Autodesk Fusion 360 part; units mm, degrees
sketch "Sketch1" plane through (0, 0, 0) normal (0, 0, 1) x (1, 0, 0)
  circle A0 centre (0, 0) radius 0.975
  dimension "d1" = 1.95
extrude "Extrude1" add sketch "Sketch1" along normal blind 6
sketch "Sketch2" plane through (0, 0, 0) normal (0, 0, -1) x (1, 0, 0)
  circle A0 centre (0, 0) radius 0.975
  circle A1 centre (0, 0) radius 1.75
  dimension "d4" = 3.5
extrude "Extrude2" add sketch "Sketch2" along normal blind 1.5 contours A0 | A1
extrude "Extrude3" cut 1 faces at (-0.5048, -0.8743, -1.5) along direction (0, 0, 1) blind 0.5
equation "d4 = ( 1.75 * 2 ) * 1 mm"
Design review of the part built by this model. Coordinates are the model's own, in mm. A direction names the side the tool comes from. Round coordinates to 2 decimals unless told otherwise and drop trailing zeros. Loops run counter-clockwise (first coordinate to the right, second up) from the corner with the lowest first, then second, coordinate; pieces in that order, holes last. Notation, with made-up numbers: M -33,-37.5 L -25,-37.5 A16 cw -25,-11.5 Z; hole C 5.25,21.25 d8. An arc over 180 degrees is marked long. Answer as a JSON object with one key per item and string values.
Item 1: We need section D-D on y = 1.2. Give the boundary of the cut face in (x, z), and give its area (3 significant figures).
Answer sheet:
{"outline": "M -1.27,-1 L 1.27,-1 L 1.27,0 L -1.27,0 Z", "area": "2.55 mm^2"}
Item 2: We need section A-A on x = 0. Give the boundary of the cut face in (y, z) (3 decimals), and give its area (3 significant figures).
Answer sheet:
{"outline": "M -1.75,-1 L 1.75,-1 L 1.75,0 L 0.975,0 L 0.975,6 L -0.975,6 L -0.975,0 L -1.75,0 Z", "area": "15.2 mm^2"}
Item 3: Machinability: for faces 3 (the cylindrical face through (-0.72, -0.66, 2.96)), 4 (the flat face through (0, 0, -1)), which of the approach directions +Z, -Z, +X, -X, +Y, -Y give a long, thin tool a straight path to every point of the face, cutting with its end or side? Answer none if there is none.
Answer sheet:
{"face 3": "+Z", "face 4": "-Z, +X, -X, +Y, -Y"}
Item 4: We need section C-C on z = 1.5. Give the boundary of the cut face in (x, y) (3 decimals).
Answer sheet:
{"outline": "C 0,0 d1.95"}
Item 5: Clearance check with a flat-ended pin moving along its axis: P1, Ø1.5, axis at x = 1.5, z = 0, coming from the +Y side. State where the tip first meets the part, or that it passes through.
Answer sheet:
{"P1": "stops at y = 1.58"}
Item 6: Wall thickness on L1, parallel to Z at x = 0.65, y = -0.9; L2, parallel to X at y = 1.3, z = -0.25; L3, parallel to X at y = 0.5, z = 3.5: over which ranges is each line inside the solid? List them lowest first. Write a range as from..to.
Answer sheet:
{"L1": "z = -1..0", "L2": "x = -1.17..1.17", "L3": "x = -0.84..0.84"}
Item 7: The part is to be moulded in two halves that separate along X. For faces 1 (the flat face through (0, 0, 6)), 2 (the cylindrical face through (1.617, -0.67, -0.493)), say which applies: pulls with the +X half, pulls with the -X half, needs draft (parallel to the pull), parting line crosses it, or undercut.
Answer sheet:
{"face 1": "needs draft", "face 2": "parting line crosses it"}
